```python
from build123d import *


with BuildPart() as part:
    # Sketch1 → Revolve1 (revolve)
    with BuildSketch(Plane(origin=(0, 0, 0), x_dir=(0, 0, -1), z_dir=(1, 0, 0)), mode=Mode.PRIVATE) as revolve1_sk:
        with BuildLine():
            Line((20, 0), (20, 14))
            Line((20, 14), (18, 14))
            Line((18, 14), (18, 16))
            Line((18, 16), (12, 16))
            Line((12, 16), (12, 14))
            Line((12, 14), (10, 14))
            ThreePointArc((10, 14), (9.324264635, 16.371708245), (7.5, 18.031128874))
            Line((7.5, 18.031128874), (0, 35))
            Line((0, 35), (0, 38.5))
            Line((0, 38.5), (-2, 38.5))
            Line((-2, 38.5), (-2, 30))
            ThreePointArc((-2, 30), (0.078015449, 18.119640862), (6.065310471, 7.65))
            Line((6.065310471, 7.65), (4.065310471, 7.65))
            Line((4.065310471, 7.65), (4.065310471, 0))
            Line((4.065310471, 0), (20, 0))
        make_face()
    revolve(revolve1_sk.sketch.rotate(Axis((0, 0, -4.065310471), (0, 0, -1)), 90), axis=Axis((0, 0, -4.065310471), (0, 0, -1)))


solid = part.part
```
The model under review builds one solid part; all positions refer to its coordinate system, in mm. A direction names the side the tool comes from. Round coordinates to 2 decimals unless told otherwise and drop trailing zeros. Order: outer loops, then holes, each group sorted by start corner. A loop starts at its lowest first (then second) coordinate and runs counter-clockwise, first axis right, second up. Notation, with made-up numbers: (87, 82) - (145, 82) arc R17 cw to (145, 102) - close; hole circle Ø6 at (-25, 16.5). An arc over 180 degrees is marked (long way). Answer in a Markdown table with one row per item.
(1) Machinability: for faces 1 (the face through (-3.47, 15.62, -14.96)), 2 (the face through (-30.55, 23.43, 1.01)), 3 (the face through (-0.07, 14.15, -12)), which of the approach directions +Z, -Z, +X, -X, +Y, -Y give a long, thin tool a straight path to every point of the face, cutting with its end or side? Answer none if there is none.
Result set:
| item | result |
|---|---|
| face 1 | -Z |
| face 2 | +Z, -Z |
| face 3 | none |
(2) For line 1 (Z direction, x = -3.5, y = 35); line 2 (X direction, y = -1.5, z = -4); line 3 (Y direction, x = -2.5, z = -4.5), list the stretches that pass through material, from the lowest coordinate up. Write a range as from..to.
Result set:
| item | result |
|---|---|
| line 1 | z = 0..2 |
| line 2 | x = -25.91..-10.3, 10.3..25.91 |
| line 3 | y = -24.69..-9.36, -7.23..7.23, 9.36..24.69 |
(3) Mouldability with a two-part tool opening along X and no side actions: class faces 4 (the face through (0, 0, -4.065)), 5 (the face through (6.5, 12.4, -19)), 6 (the face through (0, 0, -20)) as released by +X, released by -X, zero draft, split by the parting line, or undercut.
Result set:
| item | result |
|---|---|
| face 4 | undercut |
| face 5 | split by the parting line |
| face 6 | zero draft |
(4) Take a section at A-A on z = -16.5. Write out the cut boundary in (x, y).
Result set:
| item | result |
|---|---|
| outline | circle Ø32 at (0, 0) |
(5) Clearance check with flat-ended pins moving along their axes: P1, Ø7.5, axis at x = 3, y = -3, coming from the +Z side; P2, Ø9.5, axis at x = 1, y = -6, coming from the +Z side; P3, Ø4, axis at y = -13, z = -13, coming from the +X side; P4, Ø23, axis at x = -16, y = 1.5, coming from the -Z side. State where each tip first meets the part, or that it passes through.
Result set:
| item | result |
|---|---|
| P1 | stops at z = -4.07 |
| P2 | stops at z = -3.71 |
| P3 | stops at x = 11.62 |
| P4 | stops at z = -20 |
